Here's how the part is built. I have some questions about the finished solid (model axes, mm). A direction names the side the tool comes from. Round coordinates to 2 decimals unless told otherwise and drop trailing zeros. Write each loop counter-clockwise with the first axis right and the second up, starting at its lowest first coordinate (ties: lowest second). Pieces come first, ordered by that corner, then holes. Notation, with made-up numbers: (13.5, 70.5) -> (68.5, 70.5) arc R12 cw to (68.5, 80.5) -> close; hole circle Ø2 at (-14, 31.5). An arc over 180 degrees is marked (long way). Answer as CSV lines item,"result".
```python
from build123d import *

# Parameters (mm, degrees)
CROQUIS1_W              = 127
CROQUIS1_H              = 64
SALIENTE_EXTRUIR1_DEPTH = 52
CORTAR_EXTRUIR1_DEPTH   = 105.078095678
CORTAR_EXTRUIR2_DEPTH   = 105.078095678
CROQUIS4_W              = 5
CROQUIS4_H              = 20
CORTAR_EXTRUIR3_DEPTH   = 40
SALIENTE_EXTRUIR2_DEPTH = 26
VACIADO1_START          = -29.5
VACIADO1_DEPTH          = 59
VACIADO1_START_2        = 29.5
VACIADO1_2_OUTLINE_W    = 35
VACIADO1_2_OUTLINE_H    = 23.5
VACIADO1_2_DEPTH        = 3
VACIADO1_3_OUTLINE_W    = 5
VACIADO1_3_OUTLINE_H    = 17.5
VACIADO1_3_DEPTH        = 19
CORTAR_EXTRUIR4_DEPTH   = 127.684647847
SALIENTE_EXTRUIR3_DEPTH = 3
CROQUIS8_R              = 16
CORTAR_EXTRUIR5_DEPTH   = 10
CROQUIS9_R              = 18.5
CROQUIS9_R_2            = 16
SALIENTE_EXTRUIR4_DEPTH = 19
CROQUIS11_R             = 2.42
CORTAR_EXTRUIR6_DEPTH   = 39
CROQUIS12_W             = 93.002602727
CROQUIS12_H             = 56
CORTAR_EXTRUIR8_DEPTH   = 5
CROQUIS13_W             = 4
CROQUIS13_H             = 6
CROQUIS13_W_2           = 6
CROQUIS13_H_2           = 4
SALIENTE_EXTRUIR5_DEPTH = 6
CROQUIS14_R             = 1.5
CORTAR_EXTRUIR9_DEPTH   = 144.227092409


# Read off the part's stored shape, not the designer's step: Vaciado1
with BuildPart() as part:
    # Croquis1 → Saliente-Extruir1 (new body)
    with BuildSketch(Plane(origin=(0, 0, 0), x_dir=(1, 0, 0), z_dir=(0, 1, 0))):
        Rectangle(CROQUIS1_W, CROQUIS1_H)
    extrude(amount=SALIENTE_EXTRUIR1_DEPTH)

    # Croquis2 → Cortar-Extruir1 (cut, through all)
    with BuildSketch(Plane.XY.offset(32)):
        Polygon((-63.5, 52), (-63.5, 45), (-56.500349973, 51.999650027), align=None)
        Polygon((51.5, 20), (63.5, 20), (63.5, 52), (44.500349973, 51.999650027), (51.5, 45), align=None)
    extrude(amount=-CORTAR_EXTRUIR1_DEPTH, mode=Mode.SUBTRACT)

    # Croquis3 → Cortar-Extruir2 (cut, through all)
    with BuildSketch(Plane.XY.offset(32)):
        Polygon((-56.500349973, 51.999650027), (-56.487592612, 52.42007755), (-63.863183818, 52.643880882), (-63.863183818, 51.396655122), (-58.40187656, 51.777539568), align=None)
        Polygon((44.500349973, 51.999650027), (64.754794762, 55.7043164), (64.754794762, 48.499825013), align=None)
    extrude(amount=-CORTAR_EXTRUIR2_DEPTH, mode=Mode.SUBTRACT)

    # Croquis4 → Cortar-Extruir3 (cut)
    with BuildSketch(Plane.XY.offset(32)):
        with Locations((61, 10)):
            Rectangle(CROQUIS4_W, CROQUIS4_H)
    extrude(amount=-CORTAR_EXTRUIR3_DEPTH, mode=Mode.SUBTRACT)

    # Croquis5 → Saliente-Extruir2 (add)
    with BuildSketch(Plane.XZ):
        Polygon((44.5, 32), (44.5, 41), (43, 41), (43, 35), (6, 35), (6, 41), (4.5, 41), (4.5, 32), align=None)
    extrude(amount=-SALIENTE_EXTRUIR2_DEPTH)

    # Vaciado1 outline → Vaciado1 (cut)
    with BuildSketch(Plane.XY.offset(VACIADO1_START)):
        Polygon((56, 0), (56, 17.5), (49, 17.5), (49, 43.964466094), (43.464466094, 49.5), (-55.464466094, 49.5), (-61, 43.964466094), (-61, 0), align=None)
    extrude(amount=VACIADO1_DEPTH, mode=Mode.SUBTRACT)

    # Vaciado1 2 outline → Vaciado1 2 (cut)
    with BuildSketch(Plane.XY.offset(VACIADO1_START_2)):
        with Locations((24.5, 11.75)):
            Rectangle(VACIADO1_2_OUTLINE_W, VACIADO1_2_OUTLINE_H)
    extrude(amount=VACIADO1_2_DEPTH, mode=Mode.SUBTRACT)

    # Vaciado1 3 outline → Vaciado1 3 (cut)
    with BuildSketch(Plane.XY.offset(VACIADO1_START)):
        with Locations((58.5, 8.75)):
            Rectangle(VACIADO1_3_OUTLINE_W, VACIADO1_3_OUTLINE_H)
    extrude(amount=VACIADO1_3_DEPTH, mode=Mode.SUBTRACT)

    # Croquis6 → Cortar-Extruir4 (cut, through all)
    with BuildSketch(Plane(origin=(44.5, 0, 0), x_dir=(0, 0, -1), z_dir=(1, 0, 0))):
        Polygon((-41, 0), (-35, 22), (-35, 26), (-41, 26), align=None)
    extrude(amount=-CORTAR_EXTRUIR4_DEPTH, mode=Mode.SUBTRACT)

    # Croquis7 → Saliente-Extruir3 (add)
    with BuildSketch(Plane.XY.offset(32)):
        with BuildLine():
            Line((4.5, 26), (44.5, 26))
            ThreePointArc((44.5, 26), (24.5, 46), (4.5, 26))
        make_face()
    extrude(amount=SALIENTE_EXTRUIR3_DEPTH)

    # Croquis8 → Cortar-Extruir5 (cut)
    with BuildSketch(Plane.XY.offset(35)):
        with Locations((24.5, 26)):
            Circle(CROQUIS8_R)
    extrude(amount=-CORTAR_EXTRUIR5_DEPTH, mode=Mode.SUBTRACT)

    # Croquis9 → Saliente-Extruir4 (add)
    with BuildSketch(Plane(origin=(0, 0, 32.5), x_dir=(-1, 0, 0), z_dir=(0, 0, -1))):
        with Locations(Location((-24.5, 26, 0), (0, 0, 198.924644416))):
            Circle(CROQUIS9_R)
        with Locations(Location((-24.5, 26, 0), (0, 0, 180))):
            Circle(CROQUIS9_R_2, mode=Mode.SUBTRACT)
    extrude(amount=SALIENTE_EXTRUIR4_DEPTH)

    # Croquis11 → Cortar-Extruir6 (cut)
    with BuildSketch(Plane(origin=(6, 0, 0), x_dir=(0, 0, -1), z_dir=(1, 0, 0))):
        with Locations(Location((-19.360313857, 25.408506724, 0), (0, 0, 180))):
            Circle(CROQUIS11_R)
    extrude(amount=CORTAR_EXTRUIR6_DEPTH, mode=Mode.SUBTRACT)

    # Croquis12 → Cortar-Extruir8 (cut)
    with BuildSketch(Plane(origin=(0, 52, 0), x_dir=(1, 0, 0), z_dir=(0, 1, 0))):
        with Locations((-5.99903799, 0)):
            Rectangle(CROQUIS12_W, CROQUIS12_H)
    extrude(amount=-CORTAR_EXTRUIR8_DEPTH, mode=Mode.SUBTRACT)

    # Croquis13 → Saliente-Extruir5 (add)
    with BuildSketch(Plane.XZ.offset(-49.5)):
        with Locations((-27.999466094, 26.5)):
            Rectangle(CROQUIS13_W, CROQUIS13_H)
        with Locations((16.000533906, 26.5)):
            Rectangle(CROQUIS13_W, CROQUIS13_H)
        with Locations((16.000533906, -26.5)):
            Rectangle(CROQUIS13_W, CROQUIS13_H)
        with Locations((-27.999466094, -26.5)):
            Rectangle(CROQUIS13_W, CROQUIS13_H)
        with Locations((-52.464466094, 18)):
            Rectangle(CROQUIS13_W_2, CROQUIS13_H_2)
        with Locations((40.464466094, 18)):
            Rectangle(CROQUIS13_W_2, CROQUIS13_H_2)
        with Locations((40.464466094, -11)):
            Rectangle(CROQUIS13_W_2, CROQUIS13_H_2)
        with Locations((-52.464466094, -11)):
            Rectangle(CROQUIS13_W_2, CROQUIS13_H_2)
    extrude(amount=SALIENTE_EXTRUIR5_DEPTH)

    # Croquis14 → Cortar-Extruir9 (cut, through all)
    with BuildSketch(Plane.ZY.offset(63.5)):
        with Locations((-20, 4)):
            Circle(CROQUIS14_R)
        with Locations((21, 4)):
            Circle(CROQUIS14_R)
    extrude(amount=-CORTAR_EXTRUIR9_DEPTH, mode=Mode.SUBTRACT)


solid = part.part
```
1. For pin 1 Ø1 at (x, y) = (14, 8.5) entering from +Z; pin 2 Ø2 at (x, z) = (-28, -26) entering from -Y; pin 3 Ø2 at (x, z) = (16.5, 28) entering from -Y; pin 4 Ø6 at (x, z) = (-35.5, 32) entering from -Y, each with a flat end and sliding along its axis, tell me the tip position at first contact or that it passes through.
Numbers:
pin 1,"stops at z = 35"
pin 2,"stops at y = 43.5"
pin 3,"stops at y = 8.88"
pin 4,"stops at y = 0"
2. On a 3-axis mill with a long thin cutter (end or side, diameter ignored), from which of +Z, -Z, +X, -X, +Y, -Y can I reach the whole of each face in a straight line? I mean faces 1 (the face through (56, 20, -7)), 2 (the face through (-28, 49.5, -26)), 3 (the face through (61, 9, -20)). Say none if no direction works.
Numbers:
face 1,"+Z, -Z, +X, +Y"
face 2,"+Y"
face 3,"-Y"
3. If I drill on line 1 (Z direction, x = -22.5, y = 27); line 2 (X direction, y = 36.5, z = -19); line 3 (X direction, y = 14, z = -4.5), over which ranges is the centre line in solid material (lowest first)?
Numbers:
line 1,"z = -32 to -29.5, 29.5 to 32"
line 2,"x = -63.5 to -61, 49 to 51.5"
line 3,"x = -63.5 to -61, 56 to 58.5"
4. Suppose I cut it at B-B on x = -15.5. Please give me the cut outline in (y, z).
Numbers:
outline,"(0, -32) -> (52, -32) -> (52, -28) -> (49.5, -28) -> (49.5, -29.5) -> (0, -29.5) -> close; (0, 29.5) -> (49.5, 29.5) -> (49.5, 28) -> (52, 28) -> (52, 32) -> (0, 32) -> close"
5. Suppose I cut it at C-C on z = -20. Count the separate pieces of the cut face and the enclosed holes in it, and give its area (3 significant figures).
Numbers:
separate pieces,"4"
enclosed holes,"0"
area,"299 mm^2"
6. Suppose I cut it at D-D on x = 24.5. Please give me the cut outline in (y, z), and give its area (3 significant figures).
Numbers:
outline,"(0, -32) -> (52, -32) -> (52, -28) -> (49.5, -28) -> (49.5, -29.5) -> (0, -29.5) -> close; (0, 32.5) -> (7.5, 32.5) -> (7.5, 13.5) -> (10, 13.5) -> (10, 35) -> (0, 35) -> close; (42, 13.5) -> (44.5, 13.5) -> (44.5, 29.5) -> (49.5, 29.5) -> (49.5, 28) -> (52, 28) -> (52, 32) -> (46, 32) -> (46, 35) -> (42, 35) -> close"
area,"287 mm^2"
7. If we mould it in two halves opening along Z, with no side actions, what happens to faces 4 (the face through (-29.999, 47, 26)), 5 (the face through (61, 10, -8)), 6 (the face through (43, 6, 37))? For each: released by +Z, released by -Z, zero draft, split by the parting line, or undercut.
Numbers:
face 4,"undercut"
face 5,"released by +Z"
face 6,"zero draft"
